```python
from build123d import *

# Parameters (mm, degrees)
SKETCH1_R               = 18.25
SKETCH1_R_2             = 15.25
BOSS_EXTRUDE1_DEPTH     = 20
SKETCH2_R               = 1.5
CUT_EXTRUDE1_DEPTH      = 19.25
CUT_EXTRUDE1_DEPTH_BACK = 19.25
CHAMFER1_SIZE           = 1


with BuildPart() as part:
    # Sketch1 → Boss-Extrude1 (new body)
    with BuildSketch(Plane(origin=(0, 0, 0), x_dir=(1, 0, 0), z_dir=(0, 1, 0))):
        Circle(SKETCH1_R)
        Circle(SKETCH1_R_2, mode=Mode.SUBTRACT)
    extrude(amount=BOSS_EXTRUDE1_DEPTH)

    # Sketch2 → Cut-Extrude1 (cut, two sides)
    with BuildSketch(Plane.XY) as cut_extrude1_sk:
        with Locations((0, 10)):
            Circle(SKETCH2_R)
    extrude(amount=CUT_EXTRUDE1_DEPTH, mode=Mode.SUBTRACT)
    extrude(cut_extrude1_sk.sketch, amount=-CUT_EXTRUDE1_DEPTH_BACK, mode=Mode.SUBTRACT)

    # Chamfer1
    chamfer1_edges = [part.edges().sort_by_distance(p)[0] for p in [
        (-15.25, 20, 0),
    ]]
    chamfer(chamfer1_edges, length=CHAMFER1_SIZE)


solid = part.part
```
Could you check a few things on this model? Use its own coordinates, in mm. Round coordinates to 2 decimals unless told otherwise and drop trailing zeros. Write each loop counter-clockwise with the first axis right and the second up, starting at its lowest first coordinate (ties: lowest second). Pieces come first, ordered by that corner, then holes. Notation, with made-up numbers: M 86,49 L 117,49 A16 cw 117,58 Z; hole C 65.25,57 d1. An arc over 180 degrees is marked long. Write each question's results on one line, items separated by ' | '. Start each with the question number.
1. Thinking about a two-plate mould opening in Y: for faces 1 (the face through (-4, 0, 15)), 2 (the face through (-15, 20, 7)), 3 (the face through (-0.325, 8.536, -16.691)), which applies, +Y half, -Y half, draft (parallel to the pull), parting line (faces both ways), or undercut?
2. Imagine slicing it at B-B on x = 0. List the corners of the cut face in (y, z) for me.
3. Imagine slicing it at C-C on y = 10. List the corners of the cut face in (x, z) for me, and give its area (3 significant figures).
4. Imagine slicing it at D-D on y = 7.75. List the corners of the cut face in (x, z) for me, and give its area (3 significant figures).
5. Imagine slicing it at A-A on z = 0. List the corners of the cut face in (x, y) for me, and give its area (3 significant figures).
6. I'm going to push flat-ended pins straight in: pin 1 Ø8 at (y, z) = (4, 6.5) entering from -X; pin 2 Ø6 at (y, z) = (10.5, -3.5) entering from -X; pin 3 Ø12 at (y, z) = (9.5, -9) entering from +X. Where does each tip first touch, or does it pass through?
7. I need wall thicknesses on L1, parallel to X at y = 12.75, z = 0; L2, parallel to Y at x = 0, z = 16.55. Which ranges of each line are inside material? Lowest first, please. Write a range as from..to.
Result sheet:
1) face 1: -Y half | face 2: +Y half | face 3: undercut
2) outline: M 0,-18.25 L 8.5,-18.25 L 8.5,-15.25 L 0,-15.25 Z; M 0,15.25 L 8.5,15.25 L 8.5,18.25 L 0,18.25 Z; M 11.5,-18.25 L 20,-18.25 L 20,-16.25 L 19,-15.25 L 11.5,-15.25 Z; M 11.5,15.25 L 19,15.25 L 20,16.25 L 20,18.25 L 11.5,18.25 Z
3) outline: M -1.5,-18.19 L -1.5,-15.18 A15.25 cw -1.5,15.18 L -1.5,18.19 A18.25 ccw Z; M 1.5,-18.19 A18.25 ccw 1.5,18.19 L 1.5,15.18 A15.25 cw 1.5,-15.18 Z | area: 298 mm^2
4) outline: C 0,0 d36.5; hole C 0,0 d30.5 | area: 316 mm^2
5) outline: M -18.25,0 L -15.25,0 L -15.25,19 L -16.25,20 L -18.25,20 Z; M 15.25,0 L 18.25,0 L 18.25,20 L 16.25,20 L 15.25,19 Z | area: 119 mm^2
6) pin 1: stops at x = -18.08 | pin 2: stops at x = -18.24 | pin 3: stops at x = 18
7) L1: x = -18.25..-15.25, 15.25..18.25 | L2: y = 0..8.5, 11.5..20
